Source: CAD feature listing. Evaluate the final solid. Frame: model axes, mm. Face numbers are marked on the shaded views. A direction names the side the tool comes from. Round coordinates to 2 decimals unless told otherwise and drop trailing zeros. Order: outer loops, then holes, each group sorted by start corner. A loop starts at its lowest first (then second) coordinate and runs counter-clockwise, first axis right, second up. Notation, with made-up numbers: M 0.25,18 L 8.25,18 A18 ccw 8.25,45 Z; hole C -8.5,-28 d7. An arc over 180 degrees is marked long. Use CSV: the item, a comma, the result in double quotes. Start each with the question number.
```python
from build123d import *

# Parameters (mm, degrees)
SLIDER_START          = -14
SLIDER_DEPTH          = 28
RAIL_LIP_TOP_START    = 12
RAIL_LIP_TOP_DEPTH    = 2
RAIL_LIP_BOTTOM_START = -14
RAIL_LIP_BOTTOM_DEPTH = 2
FINGER_START          = -10
FINGER_DEPTH          = 20
JAW_START             = -10
JAW_DEPTH             = 20
GRIP_PAD_START        = -8
SK_6_W                = 22.3
SK_6_H                = 1.5
GRIP_PAD_DEPTH        = 16


with BuildPart() as part:
    # SK_1 → Slider (new body)
    with BuildSketch(Plane(origin=(0, 0, 0), x_dir=(1, 0, 0), z_dir=(0, 1, 0)).offset(SLIDER_START)):
        with BuildLine():
            Line((-8.7, -6), (-1, -6))
            ThreePointArc((-1, -6), (-0.292893219, -5.707106781), (0, -5))
            Line((0, -5), (0, 5))
            ThreePointArc((0, 5), (-0.292893219, 5.707106781), (-1, 6))
            Line((-1, 6), (-8.7, 6))
            ThreePointArc((-8.7, 6), (-9.407106781, 5.707106781), (-9.7, 5))
            Line((-9.7, 5), (-9.7, -5))
            ThreePointArc((-9.7, -5), (-9.407106781, -5.707106781), (-8.7, -6))
        make_face()
    extrude(amount=SLIDER_DEPTH)

    # SK_2 → Rail_Lip_Top (add)
    with BuildSketch(Plane(origin=(0, 0, 0), x_dir=(1, 0, 0), z_dir=(0, 1, 0)).offset(RAIL_LIP_TOP_START)):
        with BuildLine():
            Line((-13.45, -6), (-10.7, -6))
            ThreePointArc((-10.7, -6), (-9.992893219, -5.707106781), (-9.7, -5))
            Line((-9.7, -5), (-9.7, 5))
            ThreePointArc((-9.7, 5), (-9.992893219, 5.707106781), (-10.7, 6))
            Line((-10.7, 6), (-13.45, 6))
            ThreePointArc((-13.45, 6), (-14.157106781, 5.707106781), (-14.45, 5))
            Line((-14.45, 5), (-14.45, -5))
            ThreePointArc((-14.45, -5), (-14.157106781, -5.707106781), (-13.45, -6))
        make_face()
    extrude(amount=RAIL_LIP_TOP_DEPTH)

    # SK_3 → Rail_Lip_Bottom (add)
    with BuildSketch(Plane(origin=(0, 0, 0), x_dir=(1, 0, 0), z_dir=(0, 1, 0)).offset(RAIL_LIP_BOTTOM_START)):
        with BuildLine():
            Line((-13.45, -6), (-10.7, -6))
            ThreePointArc((-10.7, -6), (-9.992893219, -5.707106781), (-9.7, -5))
            Line((-9.7, -5), (-9.7, 5))
            ThreePointArc((-9.7, 5), (-9.992893219, 5.707106781), (-10.7, 6))
            Line((-10.7, 6), (-13.45, 6))
            ThreePointArc((-13.45, 6), (-14.157106781, 5.707106781), (-14.45, 5))
            Line((-14.45, 5), (-14.45, -5))
            ThreePointArc((-14.45, -5), (-14.157106781, -5.707106781), (-13.45, -6))
        make_face()
    extrude(amount=RAIL_LIP_BOTTOM_DEPTH)

    # SK_4 → Finger (add)
    with BuildSketch(Plane(origin=(0, 0, 0), x_dir=(1, 0, 0), z_dir=(0, 1, 0)).offset(FINGER_START)):
        with BuildLine():
            Line((1, -2.5), (43.3, -2.5))
            ThreePointArc((43.3, -2.5), (44.007106781, -2.207106781), (44.3, -1.5))
            Line((44.3, -1.5), (44.3, 1.5))
            ThreePointArc((44.3, 1.5), (44.007106781, 2.207106781), (43.3, 2.5))
            Line((43.3, 2.5), (1, 2.5))
            ThreePointArc((1, 2.5), (0.292893219, 2.207106781), (0, 1.5))
            Line((0, 1.5), (0, -1.5))
            ThreePointArc((0, -1.5), (0.292893219, -2.207106781), (1, -2.5))
        make_face()
    extrude(amount=FINGER_DEPTH)

    # SK_5 → Jaw (add)
    with BuildSketch(Plane(origin=(0, 0, 0), x_dir=(1, 0, 0), z_dir=(0, 1, 0)).offset(JAW_START)):
        with BuildLine():
            Line((21, -6.5), (43.3, -6.5))
            ThreePointArc((43.3, -6.5), (44.007106781, -6.207106781), (44.3, -5.5))
            Line((44.3, -5.5), (44.3, -3.5))
            ThreePointArc((44.3, -3.5), (44.007106781, -2.792893219), (43.3, -2.5))
            Line((43.3, -2.5), (21, -2.5))
            ThreePointArc((21, -2.5), (20.292893219, -2.792893219), (20, -3.5))
            Line((20, -3.5), (20, -5.5))
            ThreePointArc((20, -5.5), (20.292893219, -6.207106781), (21, -6.5))
        make_face()
    extrude(amount=JAW_DEPTH)

    # SK_6 → Grip_Pad (add)
    with BuildSketch(Plane(origin=(0, 0, 0), x_dir=(1, 0, 0), z_dir=(0, 1, 0)).offset(GRIP_PAD_START)):
        with Locations((32.15, -7.25)):
            Rectangle(SK_6_W, SK_6_H)
    extrude(amount=GRIP_PAD_DEPTH)


solid = part.part
```
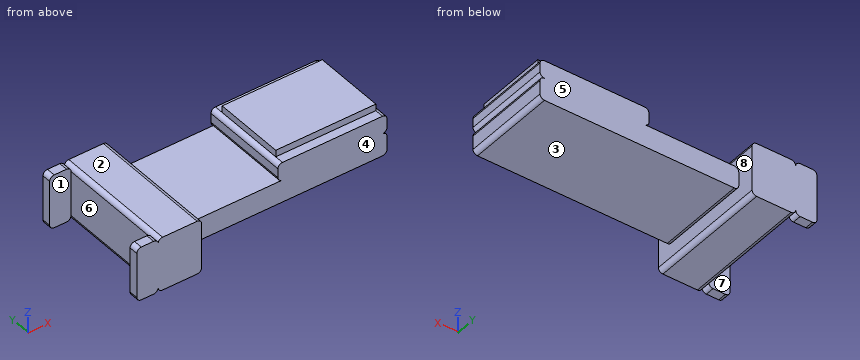
(1) Section D-D on y = 1.25. Return loops of the section in (x, z).
(2) Section B-B on x = 23. Return loops of the section in (y, z), plus the area to 3 significant figures.
(3) Draft query along X for the marked faces 6, 7 and 8. Return one class per face: pulls with the +X half, pulls with the -X half, needs draft (parallel to the pull), parting line crosses it, or undercut.
(4) Section C-C on z = 7.25. Return loops of the section in (x, y).
(5) Reachability of the marked faces 1, 2, 3, 4 and 5 from +Z, -Z, +X, -X, +Y, -Y: full face, straight path, thin tool, end or side. Return the list, or none.
(6) Contact query for flat-ended pins moving along their axis: P1, Ø2, axis at x = -7, y = -6.5, coming from the +Z side; P2, Ø3, axis at y = 5.5, z = 2.5, coming from the -X side; P3, Ø16, axis at x = 12.5, y = -4.5, coming from the +Z side. Output: stop coordinate, or through.
(7) Section A-A on y = -8.75. Return loops of the section in (x, z).
(8) Line query: line 1 along X through (y, z) = (6.5, -4.5); line 2 along X through (y, z) = (12.5, 3.25); line 3 along X through (y, z) = (-4.25, 3). Output: solid intervals per line, ascending.
Results below:
1,outline,"M -9.7,-5 A1 ccw -8.7,-6 L -1,-6 A1 ccw 0,-5 L 0,-1.5 A1 ccw 1,-2.5 L 43.3,-2.5 A1 ccw 44.3,-1.5 L 44.3,1.5 A1 ccw 43.3,2.5 A1 ccw 44.3,3.5 L 44.3,5.5 A1 ccw 43.3,6.5 L 43.3,8 L 21,8 L 21,6.5 A1 ccw 20,5.5 L 20,3.5 A1 ccw 21,2.5 L 1,2.5 A1 ccw 0,1.5 L 0,5 A1 ccw -1,6 L -8.7,6 A1 ccw -9.7,5 Z"
2,outline,"M -10,-2.5 L 10,-2.5 L 10,6.5 L 8,6.5 L 8,8 L -8,8 L -8,6.5 L -10,6.5 Z"
2,area,"204 mm2"
3,face 6,"pulls with the -X half"
3,face 7,"needs draft"
3,face 8,"undercut"
4,outline,"M 21,-8 L 43.3,-8 L 43.3,8 L 21,8 Z"
5,face 1,"+Z, -Z, -X"
5,face 2,"+Z, -X, +Y, -Y"
5,face 3,"-Z, +X, +Y, -Y"
5,face 4,"+Z, -Z, +X, -Y"
5,face 5,"+Z, -Z, +X, +Y"
6,P1,"stops at z = 6"
6,P2,"stops at x = -9.7"
6,P3,"stops at z = 6.37"
7,outline,"M -9.7,-5 A1 ccw -8.7,-6 L -1,-6 A1 ccw 0,-5 L 0,-1.5 A1 ccw 1,-2.5 L 43.3,-2.5 A1 ccw 44.3,-1.5 L 44.3,1.5 A1 ccw 43.3,2.5 A1 ccw 44.3,3.5 L 44.3,5.5 A1 ccw 43.3,6.5 L 21,6.5 A1 ccw 20,5.5 L 20,3.5 A1 ccw 21,2.5 L 1,2.5 A1 ccw 0,1.5 L 0,5 A1 ccw -1,6 L -8.7,6 A1 ccw -9.7,5 Z"
8,line 1,"x = -9.7 to 0"
8,line 2,"x = -14.45 to 0"
8,line 3,"x = -9.7 to 0, 20.13 to 44.17"
